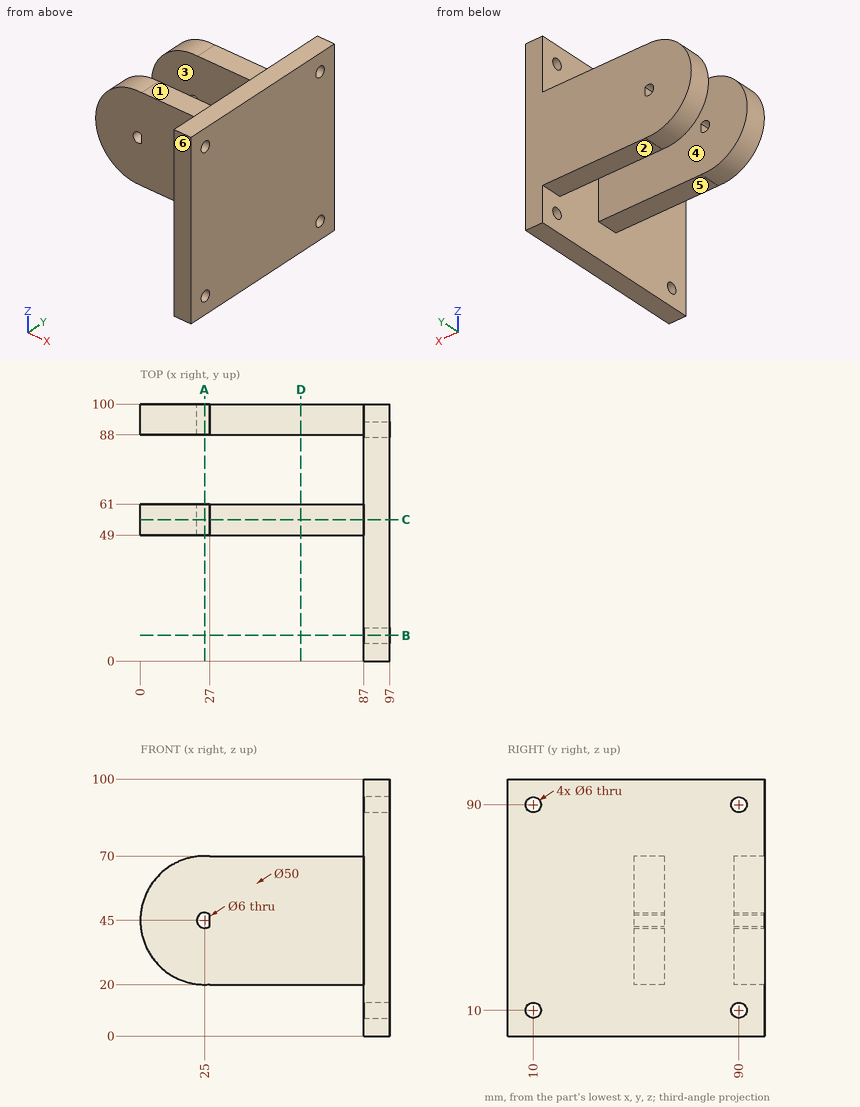
Here's the drawing with two shaded views (mm, measured from the low corner). I have some questions. A direction names the side the tool comes from. Give positions to 0.01 mm unless a question says otherwise; leave off trailing zeros. Write each loop counter-clockwise with the first axis right and the second up, starting at its lowest first coordinate (ties: lowest second). Pieces come first, ordered by that corner, then holes. Notation, with made-up numbers: (55.25, 39.5) -> (109.25, 39.5) arc R12 ccw to (109.25, 56.5) -> close; hole circle Ø6 at (-10.75, 51.5). An arc over 180 degrees is marked (long way). Answer as a JSON object with one key per item and string values. Group by question number.
Item 1: Suppose I cut it at D-D (x = 62.5). Please give me the cut outline in (y, z).
Item 2: We'd pull the mould along Y, two halves only. Please class the marked faces 4, 5 and 6: +Y half, -Y half, draft (parallel to the pull), parting line (faces both ways), or undercut.
Item 3: Suppose I cut it at A-A (x = 25). Please give me the cut outline in (y, z), plus the area to 3 significant figures.
Item 4: For the marked faces 1, 2 and 3, which set-ups out of +Z, -Z, +X, -X, +Y, -Y let a thin tool reach every point of the face, with its end or its side?
Item 5: Suppose I cut it at C-C (y = 55). Please give me the cut outline in (x, z), plus the area to 3 significant figures.
Item 6: I'm going to push flat-ended pins straight in: P1, Ø12, axis at x = 78, z = 62, coming from the -Y side; P2, Ø1.5, axis at y = 40, z = 41.5, coming from the -X side; P3, Ø6, axis at x = 61, y = 86.5, coming from the +Z side; P4, Ø5, axis at y = 90, z = 90, coming from the +X side. Where does each tip first touch, or does it pass through?
Item 7: Suppose I cut it at B-B (y = 10). Please give me the cut outline in (x, z).
Item 8: Please list where these lines run through material, in increasing order: line 1 (Y direction, x = 94, z = 90); line 2 (Y direction, x = 13, z = 63); line 3 (Z direction, x = 25, y = 57). Write a range as [from, to].
Findings:
{
 "1": {"outline": "(49, 20) -> (61, 20) -> (61, 70) -> (49, 70) -> close; (88, 20) -> (100, 20) -> (100, 70) -> (88, 70) -> close"},
 "2": {"face 4": "undercut", "face 5": "draft", "face 6": "-Y half"},
 "3": {"outline": "(49, 20) -> (61, 20) -> (61, 42) -> (49, 42) -> close; (49, 48) -> (61, 48) -> (61, 70) -> (49, 70) -> close; (88, 20) -> (100, 20) -> (100, 42) -> (88, 42) -> close; (88, 48) -> (100, 48) -> (100, 70) -> (88, 70) -> close", "area": "1,060 mm²"},
 "4": {"face 1": "+Z, -X, +Y, -Y", "face 2": "-Z, -X, +Y, -Y", "face 3": "+Z, -Z, -X"},
 "5": {"outline": "(27, 20) -> (87, 20) -> (87, 0) -> (97, 0) -> (97, 100) -> (87, 100) -> (87, 70) -> (27, 70) -> (27, 69.92) arc R25 ccw (long way) to (27, 20.08) -> close; hole (27, 42.76) -> (27, 47.24) arc R3 ccw (long way) to start", "area": "5,060 mm²"},
 "6": {"P1": "stops at y = 49", "P2": "stops at x = 87", "P3": "stops at z = 70", "P4": "passes through"},
 "7": {"outline": "(87, 0) -> (97, 0) -> (97, 7) -> (87, 7) -> close; (87, 13) -> (97, 13) -> (97, 87) -> (87, 87) -> close; (87, 93) -> (97, 93) -> (97, 100) -> (87, 100) -> close"},
 "8": {"line 1": "y = [0, 7], [13, 87], [93, 100]", "line 2": "y = [49, 61], [88, 100]", "line 3": "z = [20, 42], [48, 70]"}
}
